Geometry check sheet. Reference: drawing and pictorial views, mm from the part's lowest x, y, z. A direction names the side the tool comes from. Coordinates: 2 decimals unless noted, no trailing zeros. Write each loop counter-clockwise with the first axis right and the second up, starting at its lowest first coordinate (ties: lowest second). Pieces come first, ordered by that corner, then holes. Notation, with made-up numbers: (69, -33.75) - (89, -33.75) arc R27 cw to (89, -0.75) - close; hole circle Ø11 at (28.5, 58.25). An arc over 180 degrees is marked (long way). Use one line per item in the form item = value. Start each with the question number.
(1) Material ranges on line 1 (X direction, y = 87.5, z = 51.55) (1 decimal); line 2 (Z direction, x = 10, y = 16); line 3 (X direction, y = 86, z = 44), recorded low to high. Write a range as [from, to].
(2) Sectioned sample at C-C (z = 38). Record the cut outline in (x, y).
(3) Sectioned sample at B-B (x = 28.5). Record the cut outline in (y, z), and give its area (3 significant figures).
(4) Mould release check, pull along Z, two halves, no side actions. Record for the marked faces 1, 2 and 3: released by +Z, released by -Z, zero draft, split by the parting line, or undercut.
(5) Sectioned sample at A-A (y = 87.5). Record the cut outline in (x, z) (1 decimal).
(6) Gauge pin test, flat ends, axial feed: pin 1 Ø1.5 at (y, z) = (72, 34) entering from +X; pin 2 Ø2.5 at (x, y) = (6.01, 12.5) entering from +Z; pin 3 Ø2 at (y, z) = (43.5, 51) entering from +X; pin 4 Ø10 at (x, z) = (40, 10) entering from -Y. Record the tip position at first contact, or that the pin passes through.
(7) Tool access check on the marked faces 4 and 5. Record the directions out of +Z, -Z, +X, -X, +Y, -Y that give a thin tool (end or side, any length) a straight path to the whole face; none if there is none.
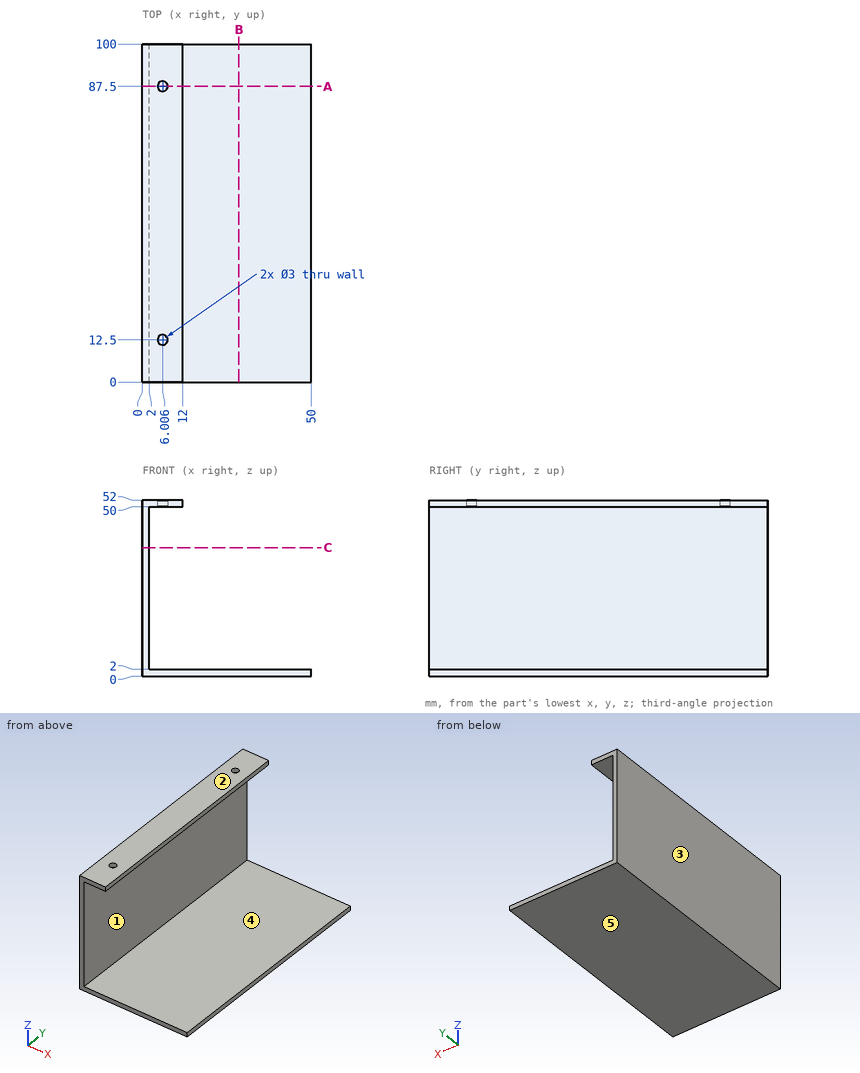
Answers below:
q1.line_1 = [0, 4.5], [7.5, 12]
q1.line_2 = [0, 2], [50, 52]
q1.line_3 = [0, 2]
q2.outline = (0, 0) - (2, 0) - (2, 100) - (0, 100) - close
q3.outline = (0, 0) - (100, 0) - (100, 2) - (0, 2) - close
q3.area = 200 mm2
q4.face_1 = undercut
q4.face_2 = released by +Z
q4.face_3 = zero draft
q5.outline = (0, 0) - (50, 0) - (50, 2) - (2, 2) - (2, 50) - (4.5, 50) - (4.5, 52) - (0, 52) - close; (7.5, 50) - (12, 50) - (12, 52) - (7.5, 52) - close
q6.pin_1 = 2
q6.pin_2 = 2
q6.pin_3 = 12
q6.pin_4 = through
q7.face_4 = +X, +Y, -Y
q7.face_5 = -Z, +X, -X, +Y, -Y
